The listing builds one solid part. Answer for the finished solid, in the listing's coordinates (mm). Face numbers are marked on the shaded views. Give positions to 0.01 mm unless a question says otherwise; leave off trailing zeros. Loops run counter-clockwise (first coordinate to the right, second up) from the corner with the lowest first, then second, coordinate; pieces in that order, holes last.
Item 1: Section C-C, the plane y = 0 is taken. Give the vertices of the cut face in (x, z), and give its area (3 significant figures).
Item 2: Section B-B, the plane x = 0 is taken. Give the vertices of the cut face in (y, z), and give its area (3 significant figures).
Item 3: This flat-tipped pin is pushed along its axis until it touches: pin 1 Ø3 at (x, y) = (-14.5, 25.5) entering from -Z. Where does it stop, or does it pass through?
Item 4: Consider line 1 along X through (y, z) = (15.5, 2.5); line 2 along Y through (x, z) = (0, 2); line 3 along X through (y, z) = (-12.5, 2). Determine where each line is inside the solid, lowest interval first.
Item 5: Section A-A, the plane x = -33 is taken. Give the vertices of the cut face in (y, z).
Item 6: Section D-D, the plane z = 3 is taken. Give the vertices of the cut face in (x, y) (3 decimals).
Item 7: The mould has two halves that part along X. Classify the marked faces 1, 2 and 3: pulls with the +X half, pulls with the -X half, needs draft (parallel to the pull), parting line crosses it, or undercut.
from build123d import *

# Parameters (mm, degrees)
SKETCH1_W           = 83
SKETCH1_H           = 65
SKETCH1_R           = 10.5
BOSS_EXTRUDE1_DEPTH = 6.5
FILLET1_R           = 5
SKETCH2_R           = 2
CUT_EXTRUDE1_DEPTH  = 10


with BuildPart() as part:
    # Sketch1 → Boss-Extrude1 (new body)
    with BuildSketch(Plane.XY):
        Rectangle(SKETCH1_W, SKETCH1_H)
        with Locations(Location((0, 0, 0), (0, 0, 180))):
            Circle(SKETCH1_R, mode=Mode.SUBTRACT)
        with BuildLine():
            Line((30.4, -18), (30.4, 18))
            ThreePointArc((30.4, 18), (33, 20.6), (35.6, 18))
            Line((35.6, 18), (35.6, -18))
            ThreePointArc((35.6, -18), (33, -20.6), (30.4, -18))
        make_face(mode=Mode.SUBTRACT)
        with BuildLine():
            Line((-30.4, -18), (-30.4, 18))
            ThreePointArc((-30.4, 18), (-33, 20.6), (-35.6, 18))
            Line((-35.6, 18), (-35.6, -18))
            ThreePointArc((-35.6, -18), (-33, -20.6), (-30.4, -18))
        make_face(mode=Mode.SUBTRACT)
    extrude(amount=BOSS_EXTRUDE1_DEPTH)

    # Fillet1
    fillet1_edges = [part.edges().sort_by_distance(p)[0] for p in [
        (-41.5, -32.5, 3.25),
        (-41.5, 32.5, 3.25),
        (41.5, 32.5, 3.25),
        (41.5, -32.5, 3.25),
    ]]
    fillet(fillet1_edges, radius=FILLET1_R)

    # Sketch2 → Cut-Extrude1 (cut)
    with BuildSketch(Plane.XY.offset(6.5)):
        with Locations((0, 27.15)):
            Circle(SKETCH2_R)
        with Locations((23.512589713, -13.575)):
            Circle(SKETCH2_R)
        with Locations((-23.512589713, -13.575)):
            Circle(SKETCH2_R)
    extrude(amount=-CUT_EXTRUDE1_DEPTH, mode=Mode.SUBTRACT)


solid = part.part
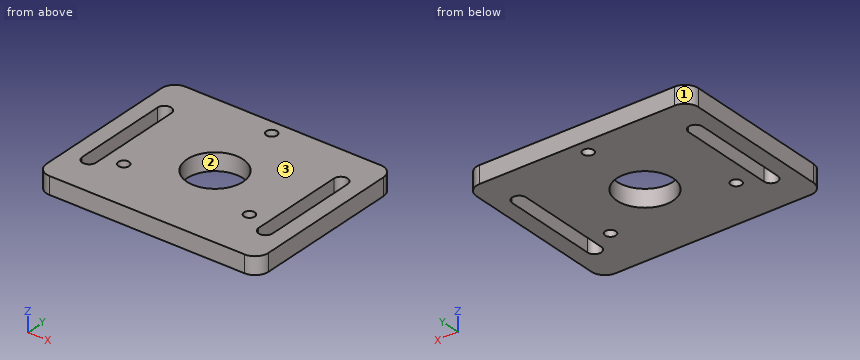
Worked answers:
1. outline: (-41.5, 0) - (-35.6, 0) - (-35.6, 6.5) - (-41.5, 6.5) - close; (-30.4, 0) - (-10.5, 0) - (-10.5, 6.5) - (-30.4, 6.5) - close; (10.5, 0) - (30.4, 0) - (30.4, 6.5) - (10.5, 6.5) - close; (35.6, 0) - (41.5, 0) - (41.5, 6.5) - (35.6, 6.5) - close
1. area: 335 mm2
2. outline: (-32.5, 0) - (-10.5, 0) - (-10.5, 6.5) - (-32.5, 6.5) - close; (10.5, 0) - (25.15, 0) - (25.15, 6.5) - (10.5, 6.5) - close; (29.15, 0) - (32.5, 0) - (32.5, 6.5) - (29.15, 6.5) - close
2. area: 260 mm2
3. pin 1: stops at z = 0
4. line 1: x = -41.5 to -35.6, -30.4 to 30.4, 35.6 to 41.5
4. line 2: y = -32.5 to -10.5, 10.5 to 25.15, 29.15 to 32.5
4. line 3: x = -41.5 to -35.6, -30.4 to -25.2, -21.83 to 21.83, 25.2 to 30.4, 35.6 to 41.5
5. outline: (-32.5, 0) - (-20.6, 0) - (-20.6, 6.5) - (-32.5, 6.5) - close; (20.6, 0) - (32.5, 0) - (32.5, 6.5) - (20.6, 6.5) - close
6. outline: (-41.5, -27.5) arc R5 ccw to (-36.5, -32.5) - (36.5, -32.5) arc R5 ccw to (41.5, -27.5) - (41.5, 27.5) arc R5 ccw to (36.5, 32.5) - (-36.5, 32.5) arc R5 ccw to (-41.5, 27.5) - close; hole (-35.6, -18) arc R2.6 ccw to (-30.4, -18) - (-30.4, 18) arc R2.6 ccw to (-35.6, 18) - close; hole circle Ø4 at (-23.513, -13.575); hole circle Ø21 at (0, 0); hole circle Ø4 at (0, 27.15); hole circle Ø4 at (23.513, -13.575); hole (30.4, -18) arc R2.6 ccw to (35.6, -18) - (35.6, 18) arc R2.6 ccw to (30.4, 18) - close
7. face 1: pulls with the -X half
7. face 2: undercut
7. face 3: needs draft
